Could you check a few things on this model? Use its own coordinates, in mm. Face numbers are marked on the shaded views. A direction names the side the tool comes from. Coordinates: 2 decimals unless noted, no trailing zeros. Write each loop counter-clockwise with the first axis right and the second up, starting at its lowest first coordinate (ties: lowest second). Pieces come first, ordered by that corner, then holes.
Item 1: I want a section at D-D on z = 21.5. Please give me the cut outline in (x, y), then the cut area to 3 significant figures.
Item 2: Which directions (+Z, -Z, +X, -X, +Y, -Y) give clear straight access to the entire face, cutting with the end or side of a thin tool? Please do the marked faces 4 and 5.
Item 3: I want a section at A-A on z = 14.5. Please give me the cut outline in (x, y).
Item 4: For P1, Ø1.6, axis at x = -51, y = 0.5, coming from the -Z side; P2, Ø1, axis at x = -51.5, y = -9, coming from the -Z side; P3, Ø2, axis at x = 51, z = 14.5, coming from the -Y side, each with a flat end and sliding along its axis, tell me the tip position at first contact or that it passes through.
Item 5: I want a section at C-C on y = 6. Please give me the cut outline in (x, z).
Item 6: If I drill on probe 1 along X at (y, z) = (18.5, 24.25); probe 2 along Y at (x, z) = (17, 15.75); probe 3 along Y at (x, z) = (-25, 11.5), over which ranges is the centre line in solid material (lowest first)?
Item 7: Thinking about a two-plate mould opening in Y: for the marked faces 1, 2 and 3, which applies, +Y half, -Y half, draft (parallel to the pull), parting line (faces both ways), or undercut?
Item 8: I want a section at B-B on x = -26.5. Please give me the cut outline in (y, z), then the cut area to 3 significant figures.
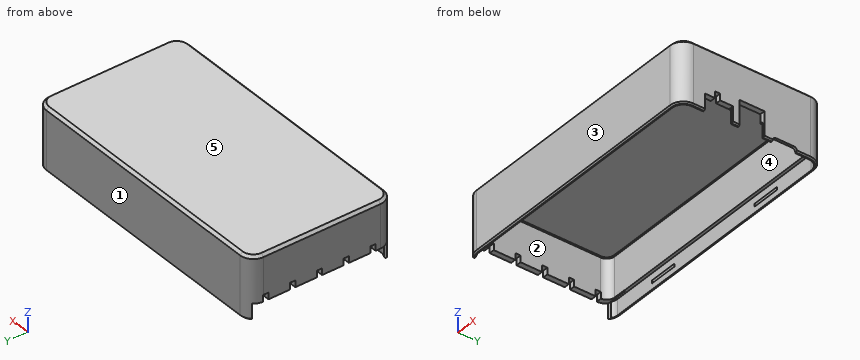
from build123d import *

# Parameters (mm, degrees)
PAD010_DEPTH                  = 23.5
POCKET028_DEPTH               = 6
PAD010_MIRRORED018_2_DEPTH    = 23.5
POCKET028_MIRRORED018_2_DEPTH = 6
PAD015_DEPTH                  = 2
PAD015_MIRRORED021_2_DEPTH    = 2
POCKET036_DEPTH               = 30.5
PAD016_DEPTH                  = 19.5
PAD016_FACE36_W               = 39
PAD016_FACE36_H               = 1.2
POCKET037_DEPTH               = 0.2
CHAMFER022_SIZE               = 0.5
CHAMFER020_SIZE               = 1
CHAMFER024_SIZE               = 0.2999
POCKET046_DEPTH               = 10
SKETCH049_W                   = 9.4
SKETCH049_H                   = 50
POCKET033_DEPTH               = 15
POCKET041_DEPTH               = 5
POCKET044_DEPTH               = 10
POCKET040_DEPTH               = 10
POCKET042_DEPTH               = 10
POCKET043_DEPTH               = 10
POCKET030_DEPTH               = 10


with BuildPart() as part:
    # Sketch033 (on DatumPlane) → Pad010 (new body)
    with BuildSketch(Plane.XY.offset(33)):
        with BuildLine():
            ThreePointArc((-47.2, 27.2), (-50.735534, 25.735534), (-52.2, 22.2))
            Line((-52.2, 0), (-52.2, 22.2))
            Line((-50.2, 0), (-52.2, 0))
            Line((-50.2, 22.2), (-50.2, 0))
            ThreePointArc((-47.2, 25.2), (-49.32132, 24.32132), (-50.2, 22.2))
            Line((0, 25.2), (-47.2, 25.2))
            Line((0, 27.2), (0, 25.2))
            Line((-47.2, 27.2), (0, 27.2))
        make_face()
    pad010 = extrude(amount=-PAD010_DEPTH)

    # Sketch031 (on Face10 of Pad010) → Pocket028 (cut)
    with BuildSketch(Plane(origin=(0, 0, 9.5), x_dir=(1, 0, 0), z_dir=(0, 0, -1))):
        with BuildLine():
            ThreePointArc((-50.2, -22.2), (-49.32132, -24.32132), (-47.2, -25.2))
            Line((-47.2, -25.2), (0, -25.2))
            Line((0, -25.2), (0, -26.3))
            Line((0, -26.3), (-47.2, -26.3))
            ThreePointArc((-51.3, -22.2), (-50.099138, -25.099138), (-47.2, -26.3))
            Line((-51.3, 0), (-51.3, -22.2))
            Line((-50.2, 0), (-51.3, 0))
            Line((-50.2, -22.2), (-50.2, 0))
        make_face()
    pocket028 = extrude(amount=-POCKET028_DEPTH, mode=Mode.SUBTRACT)

    # Sketch033 Mirrored018 2 → Pad010 Mirrored018 2 (add)
    with BuildSketch(Plane(origin=(0, 0, 33), x_dir=(-1, 0, 0), z_dir=(0, 0, -1))):
        with BuildLine():
            ThreePointArc((-47.2, 27.2), (-50.735534, 25.735534), (-52.2, 22.2))
            Line((-52.2, 0), (-52.2, 22.2))
            Line((-50.2, 0), (-52.2, 0))
            Line((-50.2, 22.2), (-50.2, 0))
            ThreePointArc((-47.2, 25.2), (-49.32132, 24.32132), (-50.2, 22.2))
            Line((0, 25.2), (-47.2, 25.2))
            Line((0, 27.2), (0, 25.2))
            Line((-47.2, 27.2), (0, 27.2))
        make_face()
    pad010_mirrored018_2 = extrude(amount=PAD010_MIRRORED018_2_DEPTH)

    # Sketch031 Mirrored018 2 → Pocket028 Mirrored018 2 (cut)
    with BuildSketch(Plane(origin=(0, 0, 9.5), x_dir=(-1, 0, 0), z_dir=(0, 0, 1))):
        with BuildLine():
            ThreePointArc((-50.2, -22.2), (-49.32132, -24.32132), (-47.2, -25.2))
            Line((-47.2, -25.2), (0, -25.2))
            Line((0, -25.2), (0, -26.3))
            Line((0, -26.3), (-47.2, -26.3))
            ThreePointArc((-51.3, -22.2), (-50.099138, -25.099138), (-47.2, -26.3))
            Line((-51.3, 0), (-51.3, -22.2))
            Line((-50.2, 0), (-51.3, 0))
            Line((-50.2, -22.2), (-50.2, 0))
        make_face()
    pocket028_mirrored018_2 = extrude(amount=POCKET028_MIRRORED018_2_DEPTH, mode=Mode.SUBTRACT)

    # Mirrored020: Pad010, Pocket028, Pad010 Mirrored018 2, Pocket028 Mirrored018 2 across Sketch033 H_Axis
    add(pad010.mirror(Plane(origin=(0, 0, 33), x_dir=(0, 0, 1), z_dir=(0, 1, 0))))
    add(pocket028.mirror(Plane(origin=(0, 0, 33), x_dir=(0, 0, 1), z_dir=(0, 1, 0))), mode=Mode.SUBTRACT)
    add(pad010_mirrored018_2.mirror(Plane(origin=(0, 0, 33), x_dir=(0, 0, 1), z_dir=(0, 1, 0))))
    add(pocket028_mirrored018_2.mirror(Plane(origin=(0, 0, 33), x_dir=(0, 0, 1), z_dir=(0, 1, 0))), mode=Mode.SUBTRACT)

    # Sketch044 (on DatumPlane) → Pad015 (join)
    with BuildSketch(Plane.XY.offset(33)):
        with BuildLine():
            ThreePointArc((-47.2, 25.2), (-49.32132, 24.32132), (-50.2, 22.2))
            Line((-50.2, 22.2), (-50.2, 0))
            Line((-50.2, 0), (0, 0))
            Line((0, 0), (0, 25.2))
            Line((0, 25.2), (-47.2, 25.2))
        make_face()
    pad015 = extrude(amount=-PAD015_DEPTH)

    # Sketch044 Mirrored021 2 → Pad015 Mirrored021 2 (add)
    with BuildSketch(Plane(origin=(0, 0, 33), x_dir=(-1, 0, 0), z_dir=(0, 0, -1))):
        with BuildLine():
            ThreePointArc((-47.2, 25.2), (-49.32132, 24.32132), (-50.2, 22.2))
            Line((-50.2, 22.2), (-50.2, 0))
            Line((-50.2, 0), (0, 0))
            Line((0, 0), (0, 25.2))
            Line((0, 25.2), (-47.2, 25.2))
        make_face()
    pad015_mirrored021_2 = extrude(amount=PAD015_MIRRORED021_2_DEPTH)

    # Mirrored027: Pad015, Pad015 Mirrored021 2 across Sketch044 H_Axis
    add(pad015.mirror(Plane(origin=(0, 0, 33), x_dir=(0, 0, 1), z_dir=(0, 1, 0))))
    add(pad015_mirrored021_2.mirror(Plane(origin=(0, 0, 33), x_dir=(0, 0, 1), z_dir=(0, 1, 0))))

    # Sketch055 → Pocket036 (cut, symmetric)
    with BuildSketch(Plane.YZ):
        with BuildLine():
            ThreePointArc((-26.1, 12.9), (-26.7, 12.3), (-26.1, 11.7))
            Line((-26.1, 12.9), (-26.1, 11.7))
        make_face()
    pocket036 = extrude(amount=POCKET036_DEPTH, both=True, mode=Mode.SUBTRACT)

    # Sketch055 → Pad016 (join, symmetric)
    with BuildSketch(Plane.YZ):
        with BuildLine():
            ThreePointArc((-26.1, 12.9), (-26.7, 12.3), (-26.1, 11.7))
            Line((-26.1, 12.9), (-26.1, 11.7))
        make_face()
    pad016 = extrude(amount=PAD016_DEPTH, both=True)

    # Pad016 Face36 → Pocket037 (cut)
    with BuildSketch(Plane(origin=(0, -26.1, 12.3), x_dir=(1, 0, 0), z_dir=(0, 1, 0))):
        Rectangle(PAD016_FACE36_W, PAD016_FACE36_H)
    pocket037 = extrude(amount=-POCKET037_DEPTH, mode=Mode.SUBTRACT)

    # Mirrored028: Pocket036, Pad016, Pocket037 across Sketch055 V_Axis
    add(pocket036.mirror(Plane(origin=(0, 0, 0), x_dir=(1, 0, 0), z_dir=(0, 1, 0))), mode=Mode.SUBTRACT)
    add(pad016.mirror(Plane(origin=(0, 0, 0), x_dir=(1, 0, 0), z_dir=(0, 1, 0))))
    add(pocket037.mirror(Plane(origin=(0, 0, 0), x_dir=(1, 0, 0), z_dir=(0, 1, 0))), mode=Mode.SUBTRACT)

    # Chamfer022
    chamfer022_edges = [part.edges().sort_by_distance(p)[0] for p in [
        (0, -27.2, 9.5),
    ]]
    chamfer(chamfer022_edges, length=CHAMFER022_SIZE)

    # Chamfer020
    chamfer020_edges = [part.edges().sort_by_distance(p)[0] for p in [
        (0, -27.2, 33),
    ]]
    chamfer(chamfer020_edges, length=CHAMFER020_SIZE)

    # Chamfer024
    chamfer024_edges = [part.edges().sort_by_distance(p)[0] for p in [
        (50.2, 0, 31),
    ]]
    chamfer(chamfer024_edges, length=CHAMFER024_SIZE)

    # Sketch041 (on DatumPlane) → Pocket046 (cut)
    with BuildSketch(Plane.YZ.offset(52.2)):
        Polygon((-7.2, 7.6), (-7.2, 15.6), (-12.1, 15.6), (-12.1, 18.1), (-14.1, 18.1), (-14.1, 15.6), (-17.8, 15.6), (-17.8, 7.6), (-17.8, 2.6), (-7.2, 2.6), align=None)
    extrude(amount=-POCKET046_DEPTH, mode=Mode.SUBTRACT)

    # Sketch049 (on DatumPlane) → Pocket033 (cut)
    with BuildSketch(Plane.YZ.offset(52.2)):
        with Locations((0, -6)):
            Rectangle(SKETCH049_W, SKETCH049_H)
    extrude(amount=-POCKET033_DEPTH, mode=Mode.SUBTRACT)

    # Sketch056 (on DatumPlane) → Pocket041 (cut)
    with BuildSketch(Plane.YZ.offset(52.2)):
        with BuildLine():
            Line((7.9, -40.25), (7.9, 9.75))
            ThreePointArc((9.15, 11), (8.266117, 10.633883), (7.9, 9.75))
            Line((9.15, 11), (15.85, 11))
            ThreePointArc((17.1, 9.75), (16.733883, 10.633883), (15.85, 11))
            Line((17.1, 9.75), (17.1, -40.25))
            Line((7.9, -40.25), (17.1, -40.25))
        make_face()
    extrude(amount=-POCKET041_DEPTH, mode=Mode.SUBTRACT)

    # Sketch050 (on DatumPlane) → Pocket044 (cut)
    with BuildSketch(Plane(origin=(-52.2, 0, 0), x_dir=(0, -1, 0), z_dir=(-1, 0, 0))):
        Polygon((-15.02, 7.6), (-15.02, 15.6), (-20.32, 15.6), (-20.32, 18.1), (-22.32, 18.1), (-22.32, 15.6), (-25.62, 15.6), (-25.62, 7.6), (-25.62, -42.4), (-15.02, -42.4), align=None)
    extrude(amount=-POCKET044_DEPTH, mode=Mode.SUBTRACT)

    # Sketch046 (on DatumPlane) → Pocket040 (cut)
    with BuildSketch(Plane(origin=(-52.2, 0, 0), x_dir=(0, -1, 0), z_dir=(-1, 0, 0))):
        Polygon((-4.86, 7.6), (-4.86, 15.6), (-10.16, 15.6), (-10.16, 18.1), (-12.16, 18.1), (-12.16, 15.6), (-15.46, 15.6), (-15.46, 7.6), (-15.46, -42.4), (-4.86, -42.4), align=None)
    extrude(amount=-POCKET040_DEPTH, mode=Mode.SUBTRACT)

    # Sketch057 (on DatumPlane) → Pocket042 (cut)
    with BuildSketch(Plane(origin=(-52.2, 0, 0), x_dir=(0, -1, 0), z_dir=(-1, 0, 0))):
        Polygon((5.3, 7.6), (5.3, 15.6), (0, 15.6), (0, 18.1), (-2, 18.1), (-2, 15.6), (-5.3, 15.6), (-5.3, 7.6), (-5.3, -42.4), (5.3, -42.4), align=None)
    extrude(amount=-POCKET042_DEPTH, mode=Mode.SUBTRACT)

    # Sketch054 (on DatumPlane) → Pocket043 (cut)
    with BuildSketch(Plane(origin=(-52.2, 0, 0), x_dir=(0, -1, 0), z_dir=(-1, 0, 0))):
        Polygon((15.46, 7.6), (15.46, 15.6), (10.16, 15.6), (10.16, 18.1), (8.16, 18.1), (8.16, 15.6), (4.86, 15.6), (4.86, 7.6), (4.86, -42.4), (15.46, -42.4), align=None)
    extrude(amount=-POCKET043_DEPTH, mode=Mode.SUBTRACT)

    # Sketch039 (on DatumPlane) → Pocket030 (cut)
    with BuildSketch(Plane(origin=(-52.2, 0, 0), x_dir=(0, -1, 0), z_dir=(-1, 0, 0))):
        Polygon((25.62, 7.6), (25.62, 15.6), (20.32, 15.6), (20.32, 18.1), (18.32, 18.1), (18.32, 15.6), (15.02, 15.6), (15.02, 7.6), (15.02, -42.4), (25.62, -42.4), align=None)
    extrude(amount=-POCKET030_DEPTH, mode=Mode.SUBTRACT)


solid = part.part
Response values:
1. outline: (-52.2, -22.2) arc R5 ccw to (-47.2, -27.2) - (47.2, -27.2) arc R5 ccw to (52.2, -22.2) - (52.2, 22.2) arc R5 ccw to (47.2, 27.2) - (-47.2, 27.2) arc R5 ccw to (-52.2, 22.2) - close; hole (-50.2, -22.2) arc R3 ccw to (-47.2, -25.2) - (47.2, -25.2) arc R3 ccw to (50.2, -22.2) - (50.2, 22.2) arc R3 ccw to (47.2, 25.2) - (-47.2, 25.2) arc R3 ccw to (-50.2, 22.2) - close
1. area: 605 mm2
2. face 4: -Z
2. face 5: +Z, +X, -X, +Y, -Y
3. outline: (-50.85, -25.62) arc R5 ccw to (-47.2, -27.2) - (47.2, -27.2) arc R5 ccw to (52.2, -22.2) - (52.2, -17.8) - (51.3, -17.8) - (51.3, -22.2) arc R4.1 cw to (47.2, -26.3) - (-47.2, -26.3) arc R4.1 cw to (-49.46, -25.62) - close; (-50.85, 25.62) - (-49.46, 25.62) arc R4.1 cw to (-47.2, 26.3) - (47.2, 26.3) arc R4.1 cw to (51.3, 22.2) - (51.3, 4.7) - (52.2, 4.7) - (52.2, 22.2) arc R5 ccw to (47.2, 27.2) - (-47.2, 27.2) arc R5 ccw to start; (51.3, -7.2) - (52.2, -7.2) - (52.2, -4.7) - (51.3, -4.7) - close
4. P1: stops at z = 15.6
4. P2: stops at z = 18.1
4. P3: stops at y = -26.34
5. outline: (-52.2, 15.6) - (-50.2, 15.6) - (-50.2, 30.7) - (-49.9, 31) - (49.9, 31) - (50.2, 30.7) - (50.2, 15.5) - (51.3, 15.5) - (51.3, 9.5) - (51.7, 9.5) - (52.2, 10) - (52.2, 32) - (51.2, 33) - (-51.2, 33) - (-52.2, 32) - close
6. probe 1: x = -52.2 to -50.2, 50.2 to 52.2
6. probe 2: y = -27.2 to -25.2, 25.2 to 27.2
6. probe 3: y = -27.2 to -26.3, 26.3 to 27.2
7. face 1: +Y half
7. face 2: undercut
7. face 3: -Y half
8. outline: (-27.2, 10) - (-26.7, 9.5) - (-26.3, 9.5) - (-26.3, 11.73) arc R0.6 cw to (-26.3, 12.87) - (-26.3, 15.5) - (-25.2, 15.5) - (-25.2, 30.7) - (-24.9, 31) - (24.9, 31) - (25.2, 30.7) - (25.2, 15.5) - (26.3, 15.5) - (26.3, 12.87) arc R0.6 cw to (26.3, 11.73) - (26.3, 9.5) - (26.7, 9.5) - (27.2, 10) - (27.2, 32) - (26.2, 33) - (-26.2, 33) - (-27.2, 32) - close
8. area: 180 mm2
